For this review, use the dimensioned drawing (mm, ordinates from the lowest corner) and the shaded views. Coordinates: 2 decimals unless noted, no trailing zeros. Loops run counter-clockwise (first coordinate to the right, second up) from the corner with the lowest first, then second, coordinate; pieces in that order, holes last. Notation, with made-up numbers: M 53.25,75.25 L 90.25,75.25 A15 cw 90.25,104.25 Z; hole C 59.5,67.5 d7. An arc over 180 degrees is marked long. One line per item, written item: value.
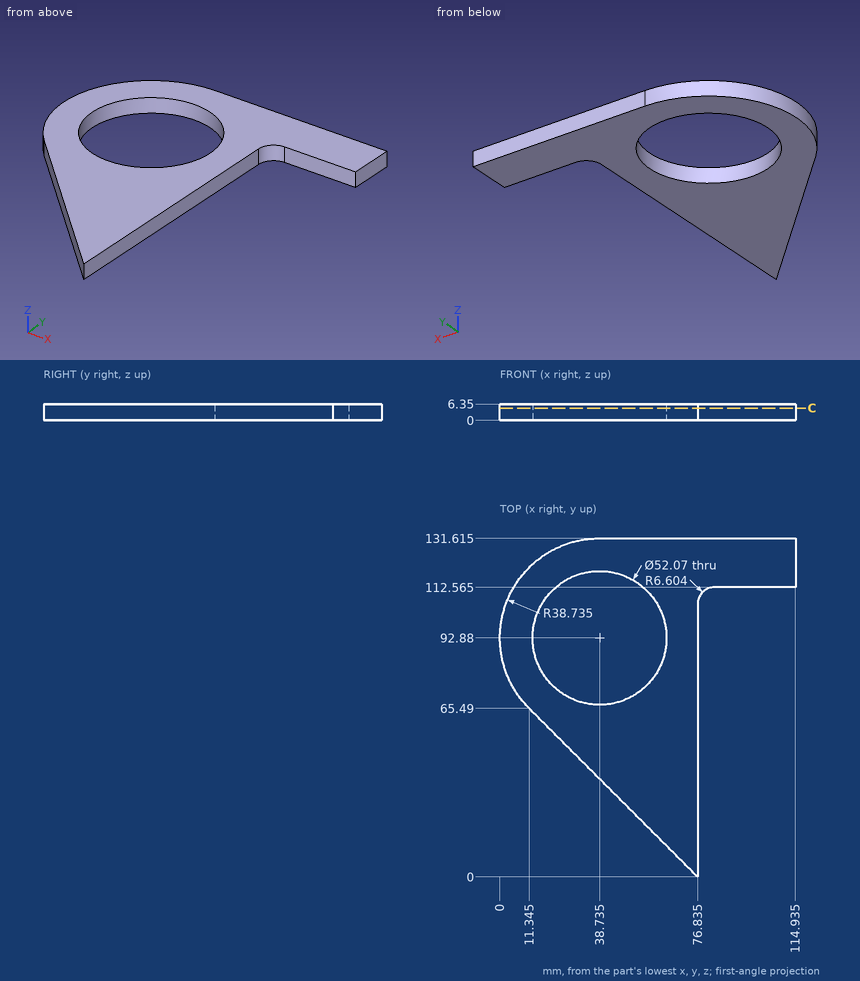
(1) We need section C-C on z = 4.75. State the section outline as (x, y) points (1 decimal), then the cut area to 3 significant figures.
Reply:
outline: M 11.3,65.5 L 76.8,0 L 76.8,106 A6.6 cw 83.4,112.6 L 114.9,112.6 L 114.9,131.6 L 38.7,131.6 A38.7 ccw Z; hole C 38.7,92.9 d52.1
area: 5,410 mm2
(2) Insertion check: pin 1 (1.5 mm diameter, centred on y = 30.5, z = 3.5, fed in from +X) (3 decimals); pin 2 (1 mm diameter, centred on y = 116.5, z = 3.5, fed in from -X); pin 3 (1.9 mm diameter, centred on x = 106.5, z = 4, fed in from -Y) (1 decimal). Each pin has a flat end and moves straight along its axis. Give the tip position at first contact, or say it passes through.
Reply:
pin 1: stops at x = 76.835
pin 2: stops at x = 7.66
pin 3: stops at y = 112.6
(3) To check wall thickness, follow line 1 along Y through (x, z) = (94.5, 2.25) (1 decimal); line 2 along Y through (x, z) = (39, 4.75) (1 decimal); line 3 along X through (y, z) = (88.5, 2.5) (1 decimal). State the ranges of each line that lie inside material, in increasing order. Write a range as [from, to].
Reply:
line 1: y = [112.6, 131.6]
line 2: y = [37.8, 66.8], [118.9, 131.6]
line 3: x = [0.2, 13.1], [64.4, 76.8]
